Part model, mm, in its own coordinate system. Coordinates: 2 decimals unless noted, no trailing zeros. Loops run counter-clockwise (first coordinate to the right, second up) from the corner with the lowest first, then second, coordinate; pieces in that order, holes last. Notation, with made-up numbers: (7.25, -34.5) -> (44.25, -34.5) arc R16 ccw to (44.25, -13.5) -> close; hole circle Ø1 at (63, 60.25). An arc over 180 degrees is marked (long way). One line per question, with ' | ' between items. Start each with the question number.
1) Cut at A-A (x = -14). List the corners of the cut face in (y, z), plus the area to 3 significant figures.
2) Cut at B-B (z = 0). List the corners of the cut face in (x, y).
3) Cut at C-C (y = -2.5). List the corners of the cut face in (x, z).
4) Probe L1, parallel to Z at x = -14, y = -2; L2, parallel to X at y = -1, z = 0; L3, parallel to X at y = -1.65, z = 3.5. List the from-to ranges inside material, lowest first. Write a range as from..to.
5) Two-plate mould, pull along X, no slides. Class faces 1 (the face through (-25.893, -2, 0)), 2 (the face through (-21.094, -2.218, -0.295)), 3 (the face through (5, -4.5, -6)): released by +X, released by -X, zero draft, split by the parting line, or undercut.
from build123d import *

# Parameters (mm, degrees)
SKETCH1_W           = 51.785459028
SKETCH1_H           = 27.470306908
BOSS_EXTRUDE1_DEPTH = 4.5


with BuildPart() as part:
    # Sketch1 → Boss-Extrude1 (new body)
    with BuildSketch(Plane(origin=(0, 0, 0), x_dir=(1, 0, 0), z_dir=(0, 1, 0))):
        Rectangle(SKETCH1_W, SKETCH1_H)
        with BuildLine():
            ThreePointArc((-7, 1.187434209), (-21.1, 0), (-7, -1.187434209))
            ThreePointArc((-7, -1.187434209), (7.1, 0), (-7, 1.187434209))
        make_face(mode=Mode.SUBTRACT)
    extrude(amount=-BOSS_EXTRUDE1_DEPTH)


solid = part.part
Reported:
1) outline: (-4.5, -13.74) -> (0, -13.74) -> (0, -7.1) -> (-4.5, -7.1) -> close; (-4.5, 7.1) -> (0, 7.1) -> (0, 13.74) -> (-4.5, 13.74) -> close | area: 59.7 mm²
2) outline: (-25.89, -4.5) -> (-21.1, -4.5) -> (-21.1, 0) -> (-25.89, 0) -> close; (7.1, -4.5) -> (25.89, -4.5) -> (25.89, 0) -> (7.1, 0) -> close
3) outline: (-25.89, -13.74) -> (25.89, -13.74) -> (25.89, 13.74) -> (-25.89, 13.74) -> close; hole (-7, -1.19) arc R7.1 ccw (long way) to (-7, 1.19) arc R7.1 ccw (long way) to start
4) L1: z = -13.74..-7.1, 7.1..13.74 | L2: x = -25.89..-21.1, 7.1..25.89 | L3: x = -25.89..-20.18, -7.82..-6.18, 6.18..25.89
5) face 1: released by -X | face 2: undercut | face 3: zero draft
